CAD build for the part. Positions are in the model's coordinates, mm. Give positions to 0.01 mm unless a question says otherwise; leave off trailing zeros. Loops run counter-clockwise (first coordinate to the right, second up) from the corner with the lowest first, then second, coordinate; pieces in that order, holes last. Notation, with made-up numbers: M -7.5,21.5 L 16.5,21.5 A16 cw 16.5,34.5 Z; hole C 46.25,-7 d8. An arc over 180 degrees is marked long. One line per question, with ' | ' between items.
```python
from build123d import *

# Parameters (mm, degrees)
F1_R     = 7.8105
F2_DEPTH = 38.1
F3_DEPTH = 50.8
F4_R     = 12.7
F4_R_2   = 7.8105
F5_DEPTH = 5.08


# Not quite as in the source:
# - a fillet or chamfer that OpenCascade refuses, or shapes differently, is made with other operations: its cross-section is extruded or revolved along the edge and cut away or added


with BuildPart() as f2:
    # F1 (on Top) → F2 (new body)
    with BuildSketch(Plane.XY):
        Circle(F1_R)
    extrude(amount=F2_DEPTH)

    # F0 (on Top) → F3 (cut)
    with BuildSketch(Plane.XY):
        with BuildLine():
            Line((-2.55, 1.8493242009), (-2.55, -1.8493242009))
            ThreePointArc((-2.55, -1.8493242009), (3.15, 0), (-2.55, 1.8493242009))
        make_face()
    extrude(amount=F3_DEPTH, mode=Mode.SUBTRACT)

    # F4 (on face) → F5 (join)
    with BuildSketch(Plane.XY.offset(38.1)):
        Circle(F4_R)
        Circle(F4_R_2, mode=Mode.SUBTRACT)
        Circle(F4_R_2)
        with BuildLine():
            Line((-2.55, -1.8493242009), (-2.55, 1.8493242009))
            ThreePointArc((-2.55, 1.8493242009), (3.15, 0), (-2.55, -1.8493242009))
        make_face(mode=Mode.SUBTRACT)
    extrude(amount=F5_DEPTH)

    # F6: chamfer of 5.08 on 1 edges, made by hand

    # F6_s1 → F6_t2 (revolve, cut)
    with BuildSketch(Plane.XZ):
        Polygon((7.8105, 5.08), (2.7305, 0), (7.8105, 0), align=None)
    revolve(axis=Axis((0, 0, 0), (0, 0, 1)), mode=Mode.SUBTRACT)


solid = f2.part
```
Item 1: Saw through at C-C on z = 25.5. Give the cut face in (x, y).
Conclusion:
outline: C 0,0 d15.62; hole M -2.55,-1.85 A3.15 ccw long -2.55,1.85 Z
Item 2: Saw through at B-B on y = 0. Give the cut face in (x, z).
Conclusion:
outline: M -12.7,38.1 L -7.81,38.1 L -7.81,5.08 L -2.73,0 L -2.55,0 L -2.55,43.18 L -12.7,43.18 Z; M 3.15,0.42 L 7.81,5.08 L 7.81,38.1 L 12.7,38.1 L 12.7,43.18 L 3.15,43.18 Z
Item 3: Saw through at D-D on x = -9. Give the cut face in (y, z).
Conclusion:
outline: M -8.96,38.1 L 8.96,38.1 L 8.96,43.18 L -8.96,43.18 Z
Item 4: Drill centre lines: line 1 along Y through (x, z) = (0, 26.5); line 2 along Z through (x, y) = (9, 3.25); line 3 along Y through (x, z) = (-1.5, 3). Where is each one in solid material? Low to high. Write a range as [from, to].
Conclusion:
line 1: [-7.81, -3.15], [3.15, 7.81] | line 2: [38.1, 43.18] | line 3: [-5.53, -2.77], [2.77, 5.53]
Item 5: Saw through at A-A on x = 0. Give the cut face in (y, z), and give its area (3 significant figures).
Conclusion:
outline: M -12.7,38.1 L -7.81,38.1 L -7.81,5.08 L -3.15,0.42 L -3.15,43.18 L -12.7,43.18 Z; M 3.15,0.42 L 7.81,5.08 L 7.81,38.1 L 12.7,38.1 L 12.7,43.18 L 3.15,43.18 Z | area: 427 mm²
Item 6: Drop flat-ended pins along their axis: P1, Ø5, axis at x = 8, z = 35.5, coming from the +Y side; P2, Ø4, axis at x = -6.5, y = 6.5, coming from the -Z side; P3, Ø12, axis at x = 7.5, z = 27.5, coming from the +Y side; P4, Ø5, axis at x = 0, y = 0, coming from the +Z side. Give the stop position or say it passes through.
Conclusion:
P1: y = 5.55 | P2: z = 4.46 | P3: y = 7.67 | P4: through
Item 7: Mould opens along Z. For faces 1 (the flat face through (5.5, 5.8, 38.1)), 2 (the flat face through (-3, 0, 43.18)), 3 (the cylindrical face through (-2.75, -12.4, 40.6)) say: pulls with the +Z half, pulls with the -Z half, needs draft (parallel to the pull), parting line crosses it, or undercut.
Conclusion:
face 1: pulls with the -Z half | face 2: pulls with the +Z half | face 3: needs draft
